Verification items for the finished model (mm, model axes). A direction names the side the tool comes from. Coordinates: 2 decimals unless noted, no trailing zeros. Order: outer loops, then holes, each group sorted by start corner. A loop starts at its lowest first (then second) coordinate and runs counter-clockwise, first axis right, second up. Notation, with made-up numbers: M 35.5,67 L 59.5,67 A18 cw 59.5,91 Z; hole C 40.5,59 d8. An arc over 180 degrees is marked long. Answer as a JSON object with one key per item and string values. Group by question number.
(1) Cross-section at D-D (z = 3.25). Enter the section's corners in (x, y).
(2) Cross-section at C-C (y = 17). Enter the section's corners in (x, z).
(3) Gauge pin test, flat ends, axial feed: pin 1 Ø0.6 at (x, z) = (5, 5) entering from +Y; pin 2 Ø7 at (x, y) = (3.5, -20) entering from +Z; pin 3 Ø3.5 at (x, y) = (-10, -10) entering from +Z; pin 4 Ø0.9 at (x, y) = (9.5, -10) entering from +Z. Record the tip position at first contact, or that the pin passes through.
(4) Cross-section at A-A (z = -2.5). Enter the section's corners in (x, y), plus the area to 3 significant figures.
(5) Cross-section at B-B (x = 2.5). Enter the section's corners in (y, z).
(6) Mould release check, pull along Y, two halves, no side actions. Record for faces 1 (the face through (0, -22.7, 1)), 2 (the face through (0, 0, 5)), 3 (the face through (10, -10, 1.5)): released by +Y, released by -Y, zero draft, split by the parting line, or undercut.
(7) Material ranges on line 1 (Y direction, x = 10, z = 4); line 2 (Y direction, x = -10, z = 4.75); line 3 (X direction, y = -10, z = 2.65), recorded low to high.
(8) Access from +Z, -Z, +X, -X, +Y, -Y to the whole of each face (thin tool, end or side, straight path). Record for faces 4 (the face through (0, 19, 4.5)), 5 (the face through (0, -19, 4.5)), 6 (the face through (6, 0, -2)), 7 (the face through (-10, -10, 1.5)).
Solid Edge part; units mm, degrees
sketch "Sketch1" plane through (0, 0, 0) normal (0, -1, 0) x (1, 0, 0)
  line L0 (-13.5, -5) -> (13.5, -5)
  line L1 (13.5, -5) -> (13.5, 5)
  line L2 (13.5, 5) -> (-13.5, 5)
  line L3 (-13.5, 5) -> (-13.5, -5)
  dimension "D1" = 13.5
  dimension "D2" = 13.5
extrude "Protrusion1" add sketch "Sketch1" along normal mid plane 45.4
sketch "Sketch2" plane through (13.5, 0, 0) normal (1, 0, 0) x (0, 1, 0)
  line L0 (-22.7, 5) -> (-16.2, 5)
  line L1 (-16.2, 5) -> (-16.2, 4.5)
  line L2 (-16.2, 4.5) -> (-22.7, 4.5)
  line L3 (-22.7, 4.5) -> (-22.7, 5)
  dimension "D1" = 22.7
extrude "Cutout1" cut sketch "Sketch2" against normal through all
mirror "Mirror1" about plane through (0, 0, 0) normal (0, -1, 0) of "Cutout1"
sketch "Sketch3" plane through (0, -22.7, -0.25) normal (0, -1, 0) x (1, 0, 0)
  line L0 (0, -4.75) -> (-6, -4.75)
  line L1 (-6, -4.75) -> (-6, 0.25)
  line L2 (-6, 0.25) -> (0, 0.25)
  line L3 (0, 0.25) -> (0, -4.75)
  dimension "D1" = 6
extrude "Cutout3" cut sketch "Sketch3" against normal through all
mirror "Mirror2" about plane through (0, 0, 0) normal (-1, 0, 0) of "Cutout3"
sketch "Sketch4" plane through (0, 0, 5) normal (0, 0, 1) x (0, 1, 0)
  circle A0 centre (-10, 10) radius 1.5
  circle A1 centre (10, 10) radius 1.5
  circle A2 centre (10, -10) radius 1.5
  circle A3 centre (-10, -10) radius 1.5
  dimension "D1" = 10
  dimension "D2" = 10
extrude "ExtrudedCutout_5" cut sketch "Sketch4" against normal blind 3.5
properties material "Stainless Steel, 304"
Taken from the geometry:
{
 "1": {"outline": "M -13.5,-22.7 L 13.5,-22.7 L 13.5,22.7 L -13.5,22.7 Z; hole C -10,-10 d3; hole C -10,10 d3; hole C 10,-10 d3; hole C 10,10 d3"},
 "2": {"outline": "M -13.5,-5 L -6,-5 L -6,0 L 6,0 L 6,-5 L 13.5,-5 L 13.5,4.5 L -13.5,4.5 Z"},
 "3": {"pin 1": "stops at y = 16.2", "pin 2": "stops at z = 4.5", "pin 3": "stops at z = 5", "pin 4": "stops at z = 1.5"},
 "4": {"outline": "M -13.5,-22.7 L -6,-22.7 L -6,22.7 L -13.5,22.7 Z; M 6,-22.7 L 13.5,-22.7 L 13.5,22.7 L 6,22.7 Z", "area": "681 mm²"},
 "5": {"outline": "M -22.7,0 L 22.7,0 L 22.7,4.5 L 16.2,4.5 L 16.2,5 L -16.2,5 L -16.2,4.5 L -22.7,4.5 Z"},
 "6": {"face 1": "released by -Y", "face 2": "zero draft", "face 3": "undercut"},
 "7": {"line 1": "y = -22.7 to -11.5, -8.5 to 8.5, 11.5 to 22.7", "line 2": "y = -16.2 to -11.5, -8.5 to 8.5, 11.5 to 16.2", "line 3": "x = -13.5 to -11.5, -8.5 to 8.5, 11.5 to 13.5"},
 "8": {"face 4": "+Z, +X, -X, +Y", "face 5": "+Z, +X, -X, -Y", "face 6": "-Z, +Y, -Y", "face 7": "+Z"}
}
